Design review of the part built by this model. Coordinates are the model's own, in mm. Face numbers are marked on the shaded views. A direction names the side the tool comes from. Give positions to 0.01 mm unless a question says otherwise; leave off trailing zeros. Write each loop counter-clockwise with the first axis right and the second up, starting at its lowest first coordinate (ties: lowest second). Pieces come first, ordered by that corner, then holes. Notation, with made-up numbers: M 56.5,-24 L 71.5,-24 A20 ccw 71.5,14 Z; hole C 49,-11 d7. An arc over 180 degrees is marked long. Answer in a Markdown table with one row per item.
```python
from build123d import *

# Parameters (mm, degrees)
SKETCH_1_W          = 50
SKETCH_1_H          = 40
EXTRUDE_1_DEPTH     = 50
CUT_EXTRUDE_1_DEPTH = 69.738635424
FILLET_1_R          = 10
FILLET_2_R          = 20
SKETCH_4_R          = 10
CUT_EXTRUDE_2_DEPTH = 50


with BuildPart() as part:
    # 草圖1 → 填料-伸長1 (new body)
    with BuildSketch(Plane(origin=(0, 0, 0), x_dir=(1, 0, 0), z_dir=(0, 1, 0))):
        Rectangle(SKETCH_1_W, SKETCH_1_H)
    extrude(amount=EXTRUDE_1_DEPTH)

    # 草圖2 → 除料-伸長1 (cut, through all)
    with BuildSketch(Plane.XY.offset(20)):
        with BuildLine():
            Line((25, 50), (5, 50))
            Line((5, 50), (5, 40))
            Line((5, 40), (-15, 40))
            Line((-15, 40), (-15, 20))
            ThreePointArc((-15, 20), (-12.071067812, 12.928932188), (-5, 10))
            Line((-5, 10), (25, 10))
            Line((25, 10), (25, 50))
        make_face()
        with BuildLine():
            ThreePointArc((-12.071067812, 0), (-21.213203436, 3.786796564), (-25, 12.928932188))
            Line((-25, 12.928932188), (-25, 0))
            Line((-25, 0), (-12.071067812, 0))
        make_face()
    extrude(amount=-CUT_EXTRUDE_1_DEPTH, mode=Mode.SUBTRACT)

    # 圓角1
    fillet_1_edges = [part.edges().sort_by_distance(p)[0] for p in [
        (5, 45, -20),
        (5, 45, 20),
    ]]
    fillet(fillet_1_edges, radius=FILLET_1_R)

    # 圓角2
    fillet_2_edges = [part.edges().sort_by_distance(p)[0] for p in [
        (25, 5, -20),
        (25, 5, 20),
    ]]
    fillet(fillet_2_edges, radius=FILLET_2_R - 0.0001)  # a hair under: the kernel refuses the full size

    # 草圖4 → 除料-伸長2 (cut)
    with BuildSketch(Plane(origin=(0, 10, 0), x_dir=(1, 0, 0), z_dir=(0, 1, 0))):
        with Locations(Location((5, 0, 0), (0, 0, 180))):
            Circle(SKETCH_4_R)
    extrude(amount=-CUT_EXTRUDE_2_DEPTH, mode=Mode.SUBTRACT)


solid = part.part
```
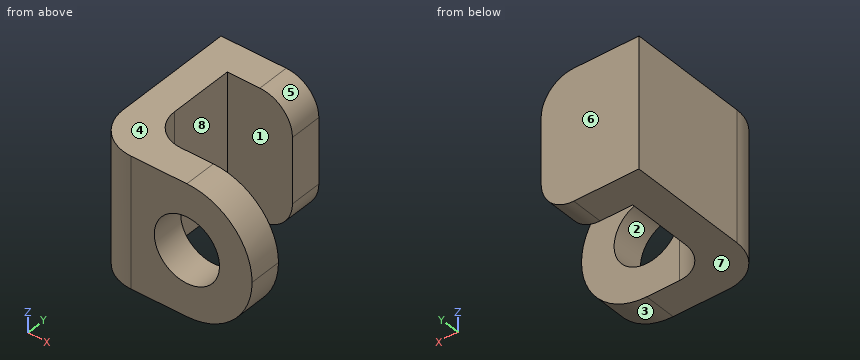
1) To check wall thickness, follow probe 1 along Z at (x, y) = (5, 7.5); probe 2 along X at (y, z) = (46.5, -3); probe 3 along Y at (x, z) = (15.5, -1). State the ranges of each line that lie inside material, in increasing order. Write a range as [from, to].
Geometry says:
| item | result |
|---|---|
| probe 1 | [-20, -10], [10, 20] |
| probe 2 | [-25, 5] |
| probe 3 | [0, 10] |
2) The part is to be moulded in two halves that separate along Y. For the marked faces 6, 7 and 8, say which applies: released by +Y, released by -Y, zero draft, split by the parting line, or undercut.
Geometry says:
| item | result |
|---|---|
| face 6 | released by +Y |
| face 7 | zero draft |
| face 8 | undercut |
3) For the marked faces 1, 2, 3, 4 and 5, list the 3-axis set-ups (+Z, -Z, +X, -X, +Y, -Y) from which the entire face can be reached by the end or side of a thin tool; tool diameter is ignored.
Geometry says:
| item | result |
|---|---|
| face 1 | +Z, -Z, +X |
| face 2 | -Y |
| face 3 | -Z, +X, +Y, -Y |
| face 4 | +Z, +X, -X, +Y, -Y |
| face 5 | +Z, +X, +Y |
4) Insertion check: P1, Ø12, axis at y = 26, z = 10.5, coming from the +X side; P2, Ø3, axis at x = 17.5, z = -3, coming from the -Y side; P3, Ø8, axis at y = 43.5, z = -0.5, coming from the +X side; P4, Ø3, axis at x = -17.5, z = 11, coming from the -Y side. Each pin has a flat end and moves straight along its axis. Give the tip position at first contact, or say it passes through.
Geometry says:
| item | result |
|---|---|
| P1 | x = -15 |
| P2 | y = 0 |
| P3 | x = 5 |
| P4 | y = 0.61 |
5) Add section A-A (x = 8.5). Write out the cut boundary in (y, z).
Geometry says:
| item | result |
|---|---|
| outline | M 0,-19.69 L 10,-19.69 L 10,-9.37 L 0,-9.37 Z; M 0,9.37 L 10,9.37 L 10,19.69 L 0,19.69 Z |
6) Add section D-D (y = 41). Write out the cut boundary in (x, z), and give its area (3 significant figures).
Geometry says:
| item | result |
|---|---|
| outline | M -25,-20 L -5,-20 A10 ccw 5,-10 L 5,10 A10 ccw -5,20 L -25,20 Z |
| area | 1,160 mm^2 |
7) Add section C-C (z = -5.5). Write out the cut boundary in (x, y).
Geometry says:
| item | result |
|---|---|
| outline | M -25,12.93 A12.93 ccw -12.07,0 L -3.35,0 L -3.35,10 L -5,10 A10 cw -15,20 L -15,40 L 5,40 L 5,50 L -25,50 Z; M 13.35,0 L 24.23,0 L 24.23,10 L 13.35,10 Z |
